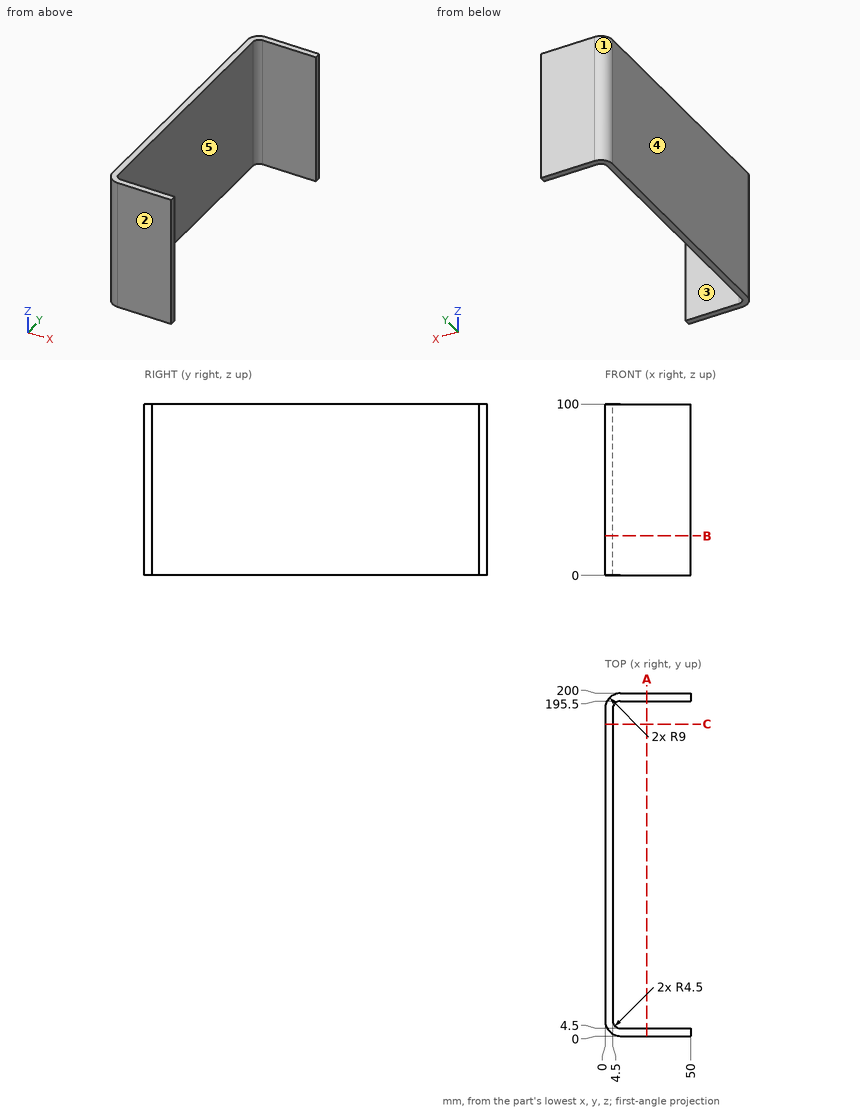
Source: three-view drawing plus pictorial views. Frame: mm from the lowest corner of the part. A direction names the side the tool comes from. Give positions to 0.01 mm unless a question says otherwise; leave off trailing zeros. Order: outer loops, then holes, each group sorted by start corner. A loop starts at its lowest first (then second) coordinate and runs counter-clockwise, first axis right, second up. Notation, with made-up numbers: (61, -25.5) - (70, -25.5) arc R35 ccw to (70, 9.5) - close; hole circle Ø10 at (67.25, 4). An arc over 180 degrees is marked (long way). Answer as a JSON object with one key per item and string values. Group by question number.
Q1. Cut plane B-B, the plane z = 23. Output: boundary loops of the cut face in (x, y), then the cut area to 3 significant figures.
Q2. Cut plane A-A, the plane x = 24.5. Output: boundary loops of the cut face in (y, z).
Q3. Cut plane C-C, the plane y = 182. Output: boundary loops of the cut face in (x, z).
Q4. First-contact query: pin 1 Ø4 at (y, z) = (111.5, 53) entering from +X. Flat tip, straight axial feed; report the tip coordinate or a pass-through.
Q5. Mould query, pull axis Y, two halves, no side actions, for the marked faces 1, 2 and 3. Classes: pulls with the +Y half, pulls with the -Y half, needs draft (parallel to the pull), parting line crosses it, or undercut.
Q6. Set-up query: the marked faces 4 and 5. Return all of +Z, -Z, +X, -X, +Y, -Y with unobstructed straight access to the full face (end or side cutting, diameter ignored); none if empty.
Q7. Line query: probe 1 along Y at (x, z) = (38.5, 50); probe 2 along X at (y, z) = (13, 7.5); probe 3 along Y at (x, z) = (6, 89.5). Output: solid intervals per line, ascending.
Results:
{
 "1": {"outline": "(0, 9) arc R9 ccw to (9, 0) - (50, 0) - (50, 4.5) - (9, 4.5) arc R4.5 cw to (4.5, 9) - (4.5, 191) arc R4.5 cw to (9, 195.5) - (50, 195.5) - (50, 200) - (9, 200) arc R9 ccw to (0, 191) - close", "area": "1,280 mm^2"},
 "2": {"outline": "(0, 0) - (4.5, 0) - (4.5, 100) - (0, 100) - close; (195.5, 0) - (200, 0) - (200, 100) - (195.5, 100) - close"},
 "3": {"outline": "(0, 0) - (4.5, 0) - (4.5, 100) - (0, 100) - close"},
 "4": {"pin 1": "x = 4.5"},
 "5": {"face 1": "pulls with the +Y half", "face 2": "pulls with the -Y half", "face 3": "undercut"},
 "6": {"face 4": "+Z, -Z, -X, +Y, -Y", "face 5": "+Z, -Z, +X"},
 "7": {"probe 1": "0 to 4.5, 195.5 to 200", "probe 2": "0 to 4.5", "probe 3": "0.51 to 5.65, 194.35 to 199.49"}
}
